The model under review builds one solid part; all positions refer to its coordinate system, in mm. A direction names the side the tool comes from. Round coordinates to 2 decimals unless told otherwise and drop trailing zeros. Write each loop counter-clockwise with the first axis right and the second up, starting at its lowest first coordinate (ties: lowest second). Pieces come first, ordered by that corner, then holes. Notation, with made-up numbers: M 40.25,1 L 90.25,1 A30 cw 90.25,28 Z; hole C 14.25,-25.75 d2. An arc over 180 degrees is marked long. One line per item, written item: value. Start each with the question number.
1) Mouldability with a two-part tool opening along X and no side actions: class faces 4 (the face through (41.47, -61.27, 26.4)), 5 (the face through (-34.377, -4.93, -31.578)), 6 (the face through (0, 23, 6)) as +X half, -X half, draft (parallel to the pull), parting line (faces both ways), or undercut.
2) Tool access review of faces 1 (the face through (5.555, 18.066, -4.259)), 2 (the face through (-27.9, -63, -35)), 3 (the face through (27.9, -63, 35)): name each direction out of +Z, -Z, +X, -X, +Y, -Y from which nothing blocks a thin tool from reaching the whole face with its end or side.
3) Take a section at B-B, the plane z = 10. Write out the cut boundary in (x, y).
4) Wall thickness on probe 1 along Z at (x, y) = (-34.8, -5.5); probe 2 along X at (y, z) = (-131, -6); probe 3 along Y at (x, z) = (-34, -25.5): over which ranges is each line inside the solid? List them lowest first.
5) Take a section at D-D, the plane x = 18.5. Write out the cut boundary in (y, z).
6) For P1, Ø8, axis at y = -41.5, z = 34, coming from the +X side; P2, Ø10, axis at y = -101.5, z = 31, coming from the -X side; P3, Ø6, axis at x = -17, z = -2, coming from the -Y side; P4, Ø5, axis at x = 34.8, z = 34.8, coming from the -Y side, all flat-tipped, find the tip position at first contact; note any pin that passes through.
7) Take a section at A-A, the plane x = 0. Write out the cut boundary in (y, z), and give its area (3 significant figures).
8) Take a section at C-C, the plane y = -25.5. Write out the cut boundary in (x, z), and give its area (3 significant figures).
from build123d import *

# Parameters (mm, degrees)
F1_DEPTH  = 114
F2_W      = 15
F2_H      = 15
F3_DEPTH  = 104
F4_R      = 3.25
F5_DEPTH  = 10
F6_R      = 5
F7_R      = 36.5
F8_DEPTH  = 1.6
F9_R      = 7
F10_DEPTH = 35
F12_DEPTH = 25
F13_R     = 7
F14_DEPTH = 34
F16_DEPTH = 25


with BuildPart() as f1:
    # F0 (on Front) → F1 (new body)
    with BuildSketch(Plane.XZ):
        with BuildLine():
            Line((37.9, 42.9), (-37.9, 42.9))
            ThreePointArc((-37.9, 42.9), (-41.4355339059, 41.4355339059), (-42.9, 37.9))
            Line((-42.9, 37.9), (-42.9, -37.9))
            ThreePointArc((-42.9, -37.9), (-41.4355339059, -41.4355339059), (-37.9, -42.9))
            Line((-37.9, -42.9), (37.9, -42.9))
            ThreePointArc((37.9, -42.9), (41.4355339059, -41.4355339059), (42.9, -37.9))
            Line((42.9, -37.9), (42.9, 37.9))
            ThreePointArc((42.9, 37.9), (41.4355339059, 41.4355339059), (37.9, 42.9))
        make_face()
    extrude(amount=F1_DEPTH)

    # F2 (on face) → F3 (cut)
    with BuildSketch(Plane.XZ.offset(114)):
        with Locations((35.4, 35.4)):
            Rectangle(F2_W, F2_H)
        with Locations((-35.4, 35.4)):
            Rectangle(F2_W, F2_H)
        with Locations((-35.4, -35.4)):
            Rectangle(F2_W, F2_H)
        with Locations((35.4, -35.4)):
            Rectangle(F2_W, F2_H)
    extrude(amount=-F3_DEPTH, mode=Mode.SUBTRACT)

    # F4 (on face) → F5 (cut, through all)
    with BuildSketch(Plane(origin=(0, 0, 0), x_dir=(-1, 0, 0), z_dir=(0, 1, 0))):
        with Locations((34.8, 34.8)):
            Circle(F4_R)
        with Locations((-34.8, 34.8)):
            Circle(F4_R)
        with Locations((34.8, -34.8)):
            Circle(F4_R)
        with Locations((-34.8, -34.8)):
            Circle(F4_R)
    extrude(amount=-F5_DEPTH, mode=Mode.SUBTRACT)

    # F6
    f6_edges = [f1.edges().sort_by_distance(p)[0] for p in [
        (-42.9, -62, 27.9),
        (-42.9, -62, -27.9),
        (-27.9, -62, -27.9),
        (-27.9, -62, -42.9),
        (27.9, -62, -42.9),
        (-27.9, -62, 42.9),
        (27.9, -62, -27.9),
        (42.9, -62, -27.9),
        (42.9, -62, 27.9),
        (27.9, -62, 42.9),
        (27.9, -62, 27.9),
        (-27.9, -62, 27.9),
    ]]
    fillet(f6_edges, radius=F6_R)

    # F7 (on face) → F8 (join)
    with BuildSketch(Plane(origin=(0, 0, 0), x_dir=(-1, 0, 0), z_dir=(0, 1, 0))):
        Circle(F7_R)
    extrude(amount=F8_DEPTH)

    # F9 (on face) → F10 (join)
    with BuildSketch(Plane(origin=(0, 0, 0), x_dir=(-1, 0, 0), z_dir=(0, 1, 0))):
        Circle(F9_R)
    extrude(amount=F10_DEPTH)

    # F11 (on face) → F12 (cut)
    with BuildSketch(Plane(origin=(0, 35, 0), x_dir=(-1, 0, 0), z_dir=(0, 1, 0))):
        Polygon((-14.5420123405, 12.7583807334), (-14.5420123405, 6), (6, 6), (6, -12.0489969126), (13.1983235478, -12.4650839716), (13.1983235478, 12.7583807334), align=None)
    extrude(amount=-F12_DEPTH, mode=Mode.SUBTRACT)

    # F13 (on face) → F14 (join)
    with BuildSketch(Plane.XZ.offset(114)):
        Circle(F13_R)
    extrude(amount=F14_DEPTH)

    # F15 (on face) → F16 (cut)
    with BuildSketch(Plane.XZ.offset(148)):
        Polygon((-6, -11.1548621207), (-6, 6), (6, 6), (-11.2425461411, 11.0141066834), align=None)
    extrude(amount=-F16_DEPTH, mode=Mode.SUBTRACT)


solid = f1.part
Checked values:
1. face 4: +X half
1. face 5: undercut
1. face 6: draft
2. face 1: +Y
2. face 2: -Z, -X, -Y
2. face 3: +Z, +X, -Y
3. outline: M -42.9,-114 L 42.9,-114 L 42.9,0 L 35.1,0 L 35.1,1.6 L -35.1,1.6 L -35.1,0 L -42.9,0 Z
4. probe 1: z = -42.9 to -38.05, -31.55 to 31.55, 38.05 to 42.9
4. probe 2: x = -3.61 to 3.61
4. probe 3: y = -114 to 0
5. outline: M -114,-42.9 L 0,-42.9 L 0,-31.46 L 1.6,-31.46 L 1.6,31.46 L 0,31.46 L 0,42.9 L -114,42.9 Z
6. P1: stops at x = 28.83
6. P2: stops at x = -41.82
6. P3: stops at y = -114
6. P4: passes through
7. outline: M -148,-7 L -114,-7 L -114,-42.9 L 0,-42.9 L 0,-36.5 L 1.6,-36.5 L 1.6,-7 L 35,-7 L 35,6 L 10,6 L 10,7 L 1.6,7 L 1.6,36.5 L 0,36.5 L 0,42.9 L -114,42.9 L -114,7 L -123,7 L -123,6 L -148,6 Z
7. area: 10,800 mm2
8. outline: M -42.9,-22.9 A5 ccw -37.9,-27.9 L -32.9,-27.9 A5 cw -27.9,-32.9 L -27.9,-37.9 A5 ccw -22.9,-42.9 L 22.9,-42.9 A5 ccw 27.9,-37.9 L 27.9,-32.9 A5 cw 32.9,-27.9 L 37.9,-27.9 A5 ccw 42.9,-22.9 L 42.9,22.9 A5 ccw 37.9,27.9 L 32.9,27.9 A5 cw 27.9,32.9 L 27.9,37.9 A5 ccw 22.9,42.9 L -22.9,42.9 A5 ccw -27.9,37.9 L -27.9,32.9 A5 cw -32.9,27.9 L -37.9,27.9 A5 ccw -42.9,22.9 Z
8. area: 6,440 mm2
